from build123d import *

# Parameters (mm, degrees)
SKETCH_1_W          = 41
SKETCH_1_H          = 40
EXTRUDE_1_DEPTH     = 0.2
SKETCH_5_R          = 4.5
CUT_EXTRUDE_3_DEPTH = 0.2
SKETCH_6_R          = 1.5
CUT_EXTRUDE_4_DEPTH = 0.2


with BuildPart() as part:
    # 스케치1 → 보스-돌출1 (new body)
    with BuildSketch(Plane.XY):
        with Locations((20.5, 20)):
            Rectangle(SKETCH_1_W, SKETCH_1_H)
    extrude(amount=EXTRUDE_1_DEPTH)

    # 스케치5 → 컷-돌출3 (cut)
    with BuildSketch(Plane.XY.offset(0.2)):
        with Locations((20.7, 19.8)):
            Circle(SKETCH_5_R)
    extrude(amount=-CUT_EXTRUDE_3_DEPTH, mode=Mode.SUBTRACT)

    # 스케치6 → 컷-돌출4 (cut)
    with BuildSketch(Plane.XY.offset(0.2)):
        with Locations((20.7, 33.75)):
            Circle(SKETCH_6_R)
        with Locations((34.65, 33.75)):
            Circle(SKETCH_6_R)
        with Locations((34.65, 19.8)):
            Circle(SKETCH_6_R)
        with Locations((20.7, 5.85)):
            Circle(SKETCH_6_R)
        with Locations((34.65, 5.85)):
            Circle(SKETCH_6_R)
        with Locations((6.75, 5.85)):
            Circle(SKETCH_6_R)
        with Locations((6.75, 33.75)):
            Circle(SKETCH_6_R)
        with Locations((6.75, 19.8)):
            Circle(SKETCH_6_R)
    extrude(amount=-CUT_EXTRUDE_4_DEPTH, mode=Mode.SUBTRACT)


solid = part.part
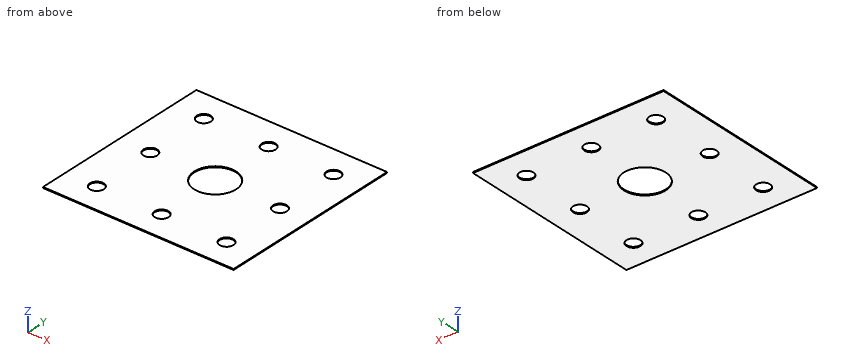
Can you work these out from the model? Positions are in its coordinate system, mm. Round coordinates to 2 decimals unless told otherwise and drop trailing zeros. Write each loop counter-clockwise with the first axis right and the second up, starting at its lowest first coordinate (ties: lowest second). Pieces come first, ordered by that corner, then holes. Notation, with made-up numbers: (-33, -22.75) -> (-16, -22.75) arc R21 ccw to (-16, -6.75) -> close; hole circle Ø5 at (32.5, 49). An arc over 180 degrees is marked (long way). Use one line per item in the form item = value. Start each with the question number.
Q1. Imagine slicing it at A-A (y = 5.85). Please give me the cut outline in (x, z).
Q2. Imagine slicing it at D-D (x = 17.5). Please give me the cut outline in (y, z), then the cut area to 3 significant figures.
Q3. Imagine slicing it at C-C (z = 0.15). Count the separate pieces of the cut face and the enclosed holes in it, then the cut area to 3 significant figures.
Q4. If I drill on probe 1 along Y at (x, z) = (20.7, 0.1); probe 2 along Y at (x, z) = (6.75, 0.1); probe 3 along Y at (x, z) = (24, 0.1), over which ranges is the centre line in solid material (lowest first)? Write a range as [from, to].
Q5. Imagine slicing it at B-B (x = 6.75). Please give me the cut outline in (y, z), then the cut area to 3 significant figures.
Q6. I'm going to push flat-ended pins straight in: P1, Ø1.8, axis at x = 6.75, y = 5.85, coming from the -Z side; P2, Ø3.5, axis at x = 6.75, y = 33.75, coming from the -Z side. Where does each tip first touch, or does it pass through?
Worked out:
q1.outline = (0, 0) -> (5.25, 0) -> (5.25, 0.2) -> (0, 0.2) -> close; (8.25, 0) -> (19.2, 0) -> (19.2, 0.2) -> (8.25, 0.2) -> close; (22.2, 0) -> (33.15, 0) -> (33.15, 0.2) -> (22.2, 0.2) -> close; (36.15, 0) -> (41, 0) -> (41, 0.2) -> (36.15, 0.2) -> close
q2.outline = (0, 0) -> (16.64, 0) -> (16.64, 0.2) -> (0, 0.2) -> close; (22.96, 0) -> (40, 0) -> (40, 0.2) -> (22.96, 0.2) -> close
q2.area = 6.73 mm^2
q3.separate_pieces = 1
q3.enclosed_holes = 9
q3.area = 1,520 mm^2
q4.probe_1 = [0, 4.35], [7.35, 15.3], [24.3, 32.25], [35.25, 40]
q4.probe_2 = [0, 4.35], [7.35, 18.3], [21.3, 32.25], [35.25, 40]
q4.probe_3 = [0, 16.74], [22.86, 40]
q5.outline = (0, 0) -> (4.35, 0) -> (4.35, 0.2) -> (0, 0.2) -> close; (7.35, 0) -> (18.3, 0) -> (18.3, 0.2) -> (7.35, 0.2) -> close; (21.3, 0) -> (32.25, 0) -> (32.25, 0.2) -> (21.3, 0.2) -> close; (35.25, 0) -> (40, 0) -> (40, 0.2) -> (35.25, 0.2) -> close
q5.area = 6.20 mm^2
q6.P1 = through
q6.P2 = 0
